```python
from build123d import *

# Parameters (mm, degrees)
BOSS_EXTRUDE1_DEPTH = 6
SKETCH2_R           = 5
CUT_EXTRUDE1_DEPTH  = 3


with BuildPart() as part:
    # Sketch1 → Boss-Extrude1 (new body)
    with BuildSketch(Plane(origin=(0, 0, 0), x_dir=(0, 1, 0), z_dir=(0, 0, 1))):
        with BuildLine():
            Line((16.223609114, -9.713238737), (9.569519391, -9.713238737))
            Line((9.569519391, -9.713238737), (19.093109625, -27.018057697))
            Line((19.093109625, -27.018057697), (13.668710041, -45.720503906))
            Line((13.668710041, -45.720503906), (8.303421987, -45.720503906))
            Line((8.303421987, -45.720503906), (10.986066014, -36.471184268))
            Line((10.986066014, -36.471184268), (12.646750412, -27.018057697))
            Line((12.646750412, -27.018057697), (3.960093563, -9.713238737))
            Line((3.960093563, -9.713238737), (-1.54802471, -9.713238737))
            Line((-1.54802471, -9.713238737), (-4.031835178, -25.485118253))
            Line((-4.031835178, -25.485118253), (1.277145856, -34.519377583))
            Line((1.277145856, -34.519377583), (-4.031835178, -45.720503906))
            Line((-4.031835178, -45.720503906), (-9.637527873, -43.063582152))
            Line((-9.637527873, -43.063582152), (-4.854308239, -32.971730814))
            Line((-4.854308239, -32.971730814), (-9.637527873, -25.485118253))
            Line((-9.637527873, -25.485118253), (-7.153717404, -9.713238737))
            Line((-7.153717404, -9.713238737), (-14.656334984, -9.713238737))
            Line((-14.656334984, -9.713238737), (-22.594802565, -22.879879476))
            Line((-22.594802565, -22.879879476), (-20.295393399, -43.063582152))
            Line((-20.295393399, -43.063582152), (-27.465165035, -43.880391579))
            Line((-27.465165035, -43.880391579), (-29.764574201, -23.696688902))
            Line((-29.764574201, -23.696688902), (-20.295393399, -9.713238737))
            ThreePointArc((-20.295393399, -9.713238737), (0, 22.5), (20.295393399, -9.713238737))
            Line((20.295393399, -9.713238737), (31.307295072, -25.485118253))
            Line((31.307295072, -25.485118253), (37.404948205, -29.824166519))
            Line((37.404948205, -29.824166519), (36.171384738, -36.030726629))
            Line((36.171384738, -36.030726629), (26.443205406, -30.722661353))
            Line((26.443205406, -30.722661353), (24.903556479, -25.485118253))
            Line((24.903556479, -25.485118253), (16.223609114, -9.713238737))
        make_face()
    extrude(amount=BOSS_EXTRUDE1_DEPTH)

    # Sketch2 → Cut-Extrude1 (cut)
    with BuildSketch(Plane(origin=(0, 0, 0), x_dir=(1, 0, 0), z_dir=(0, 0, -1))):
        with Locations(Location((0, 0, 0), (0, 0, 180))):
            Circle(SKETCH2_R)
    extrude(amount=-CUT_EXTRUDE1_DEPTH, mode=Mode.SUBTRACT)


solid = part.part
```
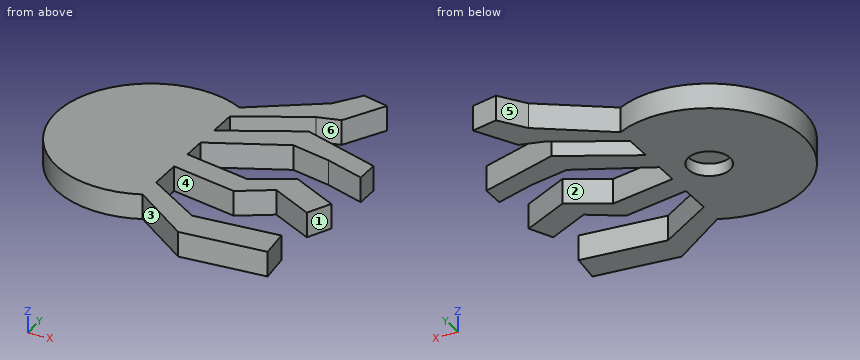
Geometry: final body of the model. Coordinates: model frame, mm. Face numbers are marked on the shaded views. A direction names the side the tool comes from. Coordinates: 2 decimals unless noted, no trailing zeros. Order: outer loops, then holes, each group sorted by start corner. A loop starts at its lowest first (then second) coordinate and runs counter-clockwise, first axis right, second up. Notation, with made-up numbers: (36.5, 3.5) -> (89.5, 3.5) arc R27 ccw to (89.5, 38.5) -> close; hole circle Ø1 at (43.25, -21). An arc over 180 degrees is marked (long way). Answer in a Markdown table with one row per item.
Item 1: Section A-A on x = 0. Output: boundary loops of the cut face in (y, z), plus the area to 3 significant figures.
Return value:
| item | result |
|---|---|
| outline | (-22.5, 0) -> (-5, 0) -> (-5, 3) -> (5, 3) -> (5, 0) -> (22.5, 0) -> (22.5, 6) -> (-22.5, 6) -> close |
| area | 240 mm² |
Item 2: Section C-C on y = 0. Output: boundary loops of the cut face in (x, z).
Return value:
| item | result |
|---|---|
| outline | (-22.5, 0) -> (-5, 0) -> (-5, 3) -> (5, 3) -> (5, 0) -> (9.71, 0) -> (9.71, 6) -> (-22.5, 6) -> close; (32.35, 0) -> (37.21, 0) -> (37.21, 6) -> (32.35, 6) -> close |
Item 3: Access query for the marked faces 1, 2 and 3. Directions: +Z, -Z, +X, -X, +Y, -Y. A direction counts if a zero-diameter tool reaches every point of the face in a straight line with its end or side. Return the directions, or none.
Return value:
| item | result |
|---|---|
| face 1 | +Z, -Z, +X |
| face 2 | +Z, -Z |
| face 3 | +Z, -Z, -Y |
Item 4: Draft query along X for the marked faces 4, 5 and 6. Return one class per face: released by +X, released by -X, zero draft, split by the parting line, or undercut.
Return value:
| item | result |
|---|---|
| face 4 | undercut |
| face 5 | released by -X |
| face 6 | released by +X |
Item 5: Ray query, L1, parallel to Y at x = 0, z = 1; L2, parallel to Y at x = 25, z = 4.5; L3, parallel to Y at x = 26.5, z = 4.25. Return the intervals inside material, ascending.
Return value:
| item | result |
|---|---|
| L1 | y = -22.5 to -5, 5 to 22.5 |
| L2 | y = -29.62 to -22.35, -9.56 to -3.96, 11.63 to 17.98, 24.64 to 30.97 |
| L3 | y = -29.45 to -22.18, -8.99 to -3.44, 12.39 to 18.81, 25.2 to 32.73 |
Item 6: Contact query for flat-ended pins moving along their axis: P1, Ø3, axis at y = 14, z = 2.5, coming from the +X side; P2, Ø1, axis at y = 5.5, z = 2.5, coming from the -X side; P3, Ø3, axis at x = -13, z = 1, coming from the -Y side; P4, Ø1.5, axis at x = 31, z = 4, coming from the -Y side. Output: stop coordinate, or through.
Return value:
| item | result |
|---|---|
| P1 | stops at x = 45.72 |
| P2 | stops at x = -21.94 |
| P3 | stops at y = -19.34 |
| P4 | stops at y = -29.02 |
Item 7: Section D-D on y = -13.5. Output: boundary loops of the cut face in (x, z), plus the area to 3 significant figures.
Return value:
| item | result |
|---|---|
| outline | (-18, 0) -> (9.71, 0) -> (9.71, 6) -> (-18, 6) -> close |
| area | 166 mm² |
